Autodesk Inventor part; units mm, degrees
ref_plane "WorkPlane1" through (0, 0, 0) normal (0, 0, 1) x (1, 0, 0)
ref_plane "Work Plane2" through (0, 0, -1) normal (0, 0, 1) x (1, 0, 0)
ref_plane "WorkPlane2" through (0, 0, 1) normal (0, 0, 1) x (1, 0, 0)
ref_plane "WorkPlane1" through (0, 0, 0) normal (0, 0, 1) x (1, 0, 0)
ref_plane "Work Plane2" through (0, 0, -1) normal (0, 0, 1) x (1, 0, 0)
ref_plane "WorkPlane2" through (0, 0, 1) normal (0, 0, 1) x (1, 0, 0)
sketch "Szkic1" plane through (0, 0, 0) normal (0, 0, 1) x (1, 0, 0)
  point P0 (0, 0)
sketch "Szkic2" plane through (0, 0, 0) normal (0, 0, 1) x (1, 0, 0)
  line L0 (5.2, -9.7072) -> (4.4019, -8.1329)
  arc A0 (6.8278, -5.7169) -> (4.4019, -8.1329) centre (6.0074, -7.319) ccw
  line L1 (6.8278, -5.7169) -> (7.8396, -6.235)
  arc A1 (7.8396, -6.235) -> (-7.8396, -6.235) centre (0, 0) ccw
  line L2 (-6.8278, -5.7169) -> (-7.8396, -6.235)
  arc A2 (-4.4019, -8.1329) -> (-6.8278, -5.7169) centre (-6.0074, -7.319) ccw
  line L3 (-5.2, -9.7072) -> (-4.4019, -8.1329)
  arc A3 (5.2, -9.7072) -> (-5.2, -9.7072) centre (0, 0.55) ccw
  line L4 (0, 0.55) -> (-5.2, -9.7072) construction
  line L5 (0, 0.55) -> (5.2, -9.7072) construction
  dimension "d2" = 11.5
  dimension "d4" = 0
  dimension "d6" = 10.0167
  dimension "d8" = 0.55
  dimension "d10" = 5.2
  dimension "d12" = 5.2
  dimension "d14" = 1.8
  dimension "d16" = 1.8
  dimension "d18" = 9.9
  dimension "d20" = 9.9
  dimension "d22" = 36
  dimension "d24" = 36
extrude "Wyciągnięcie proste1" add sketch "Szkic2" along normal blind 1
sketch "Szkic3" plane through (0, 0, 1) normal (0, 0, 1) x (1, 0, 0)
  arc A0 (-4.4019, -8.1329) -> (-6.8278, -5.7169) centre (-6.0074, -7.319) ccw
hole "Otwór1" at (-6.0074, -7.319, 1) direction (0, 0, -1) diameter 2 end through all
sketch "Szkic4" plane through (0, 0, 1) normal (0, 0, 1) x (1, 0, 0)
  arc A0 (6.8278, -5.7169) -> (4.4019, -8.1329) centre (6.0074, -7.319) ccw
hole "Otwór2" at (6.0074, -7.319, 1) direction (0, 0, -1) diameter 2 end through all
equation "\"d2\" = 0.5 * Diam2"
equation "\"d6\" = 0.5 * msp_dd1"
equation "\"d8\" = -0.5 * msp_dd1 + 0.5 * Diam2 - 0.222222 * ParA"
equation "\"d10\" = 2.6 * Diam5"
equation "\"d12\" = 2.6 * Diam5"
equation "\"d14\" = 0.9 * Diam5"
equation "\"d16\" = 0.9 * Diam5"
equation "\"d18\" = 1.3 * Diam5 + 0.5 * Diam2 - ParA"
equation "\"d20\" = 1.3 * Diam5 + 0.5 * Diam2 - ParA"
equation "\"d25\" = ParS"
equation "\"d29\" = Diam5"
equation "\"d36\" = Diam5"
equation "\"Diam5\" = 2"
equation "\"ParA\" = 4.2"
equation "\"ParS\" = 1"
equation "\"Diam2\" = 23"
equation "\"msp_dd1\" = -b + Diam2 - 0.111111 * ParA"
equation "\"msp_pom\" = 0.5 * Diam2 - b"
equation "\"TEMPLATE\" = 1.2345"
properties part number "DIN 472 - 22x1" material "Stal, miękka"
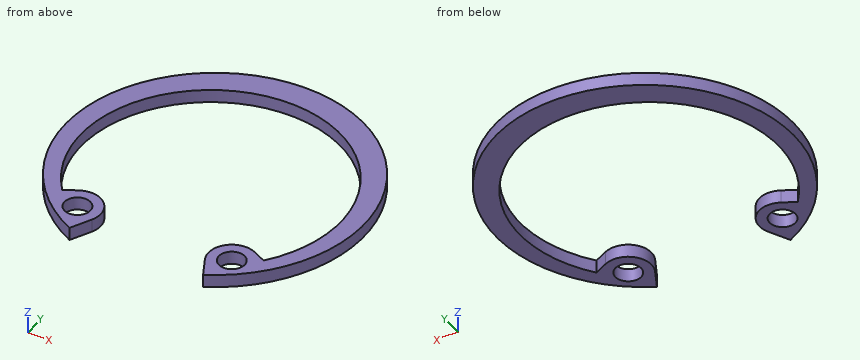
Verification items for the finished model (mm, model axes). Give positions to 0.01 mm unless a question says otherwise; leave off trailing zeros. Loops run counter-clockwise (first coordinate to the right, second up) from the corner with the lowest first, then second, coordinate; pieces in that order, holes last.
1. Section check C-C, the plane z = 0.5. Enter the section's corners in (x, y) (3 decimals).
2. Section check B-B, the plane y = 8.25. Enter the section's corners in (x, z), then the cut area to 3 significant figures.
3. Thickness scan on line 1 (Y direction, x = -6.5, z = 0.6); line 2 (Y direction, x = -5.75, z = 0.3); line 3 (Y direction, x = 0, z = 0.3). Record the ranges inside material, lowest first.
4. Section check D-D, the plane x = 0. Enter the section's corners in (y, z), then the cut area to 3 significant figures.
5. Section check A-A, the plane x = -4.75. Enter the section's corners in (y, z), then the cut area to 3 significant figures.
Geometry says:
1. outline: (-7.84, -6.235) arc R10.017 cw (long way) to (7.84, -6.235) - (6.828, -5.717) arc R1.8 ccw to (4.402, -8.133) - (5.2, -9.707) arc R11.5 ccw (long way) to (-5.2, -9.707) - (-4.402, -8.133) arc R1.8 ccw to (-6.828, -5.717) - close; hole circle Ø2 at (-6.007, -7.319); hole circle Ø2 at (6.007, -7.319)
2. outline: (-8.54, 0) - (-5.68, 0) - (-5.68, 1) - (-8.54, 1) - close; (5.68, 0) - (8.54, 0) - (8.54, 1) - (5.68, 1) - close
2. area: 5.72 mm2
3. line 1: y = -8.94 to -8.19, -6.45 to -5.59, 7.62 to 10.04
3. line 2: y = -9.41 to -8.29, -6.35 to -5.54, 8.2 to 10.51
3. line 3: y = 10.02 to 12.05
4. outline: (10.02, 0) - (12.05, 0) - (12.05, 1) - (10.02, 1) - close
4. area: 2.03 mm2
5. outline: (-8.82, 0) - (-6.03, 0) - (-6.03, 1) - (-8.82, 1) - close; (8.82, 0) - (11.02, 0) - (11.02, 1) - (8.82, 1) - close
5. area: 4.99 mm2
